Design review of the part built by this model. Coordinates are the model's own, in mm. A direction names the side the tool comes from. Coordinates: 2 decimals unless noted, no trailing zeros. Write each loop counter-clockwise with the first axis right and the second up, starting at its lowest first coordinate (ties: lowest second). Pieces come first, ordered by that corner, then holes. Notation, with made-up numbers: (69.5, 26) - (124.5, 26) arc R25 cw to (124.5, 51) - close; hole circle Ø1 at (-32, 84). An arc over 180 degrees is marked (long way). One line per item, written item: value.
from build123d import *

# Parameters (mm, degrees)
SKETCH_1_W          = 2
SKETCH_1_H          = 7
EXTRUDE_2_DEPTH     = 7
FILLET_1_R          = 3.5
SKETCH_2_R          = 1.55
CUT_EXTRUDE_1_DEPTH = 17.408839081
SKETCH_3_W          = 3.5
SKETCH_3_H          = 3
EXTRUDE_4_DEPTH     = 7
FILLET_2_R          = 3.5
SKETCH_4_R          = 1.5
CUT_EXTRUDE_2_DEPTH = 15.230249471
FILLET_3_R          = 3.5
FILLET_4_R          = 1.5
FILLET_5_R          = 0.8


# Some blends are built 0.0001 mm under size
with BuildPart() as part:
    # 草图1 → 凸台-拉伸2 (new body)
    with BuildSketch(Plane(origin=(0, 0, 0), x_dir=(1, 0, 0), z_dir=(0, 1, 0))):
        Polygon((-3.5, -3.5), (-3.5, 3.5), (-0.5, 3.5), (-0.5, 5.5), (-2.5, 5.5), (-5.5, 5.5), (-5.5, -5.5), (5.5, -5.5), (5.5, 5.5), (2.5, 5.5), (0.5, 5.5), (0.5, 3.5), (3.5, 3.5), (3.5, -3.5), align=None)
        with Locations((-1.5, 9)):
            Rectangle(SKETCH_1_W, SKETCH_1_H)
        with Locations((1.5, 9)):
            Rectangle(SKETCH_1_W, SKETCH_1_H)
    extrude(amount=EXTRUDE_2_DEPTH)

    # 圆角1
    fillet_1_edges = [part.edges().sort_by_distance(p)[0] for p in [
        (1.5, 7, -12.5),
        (1.5, 0, -12.5),
        (-1.5, 0, -12.5),
        (-1.5, 7, -12.5),
    ]]
    fillet(fillet_1_edges, radius=FILLET_1_R - 0.0001)  # a hair under: the kernel refuses the full size

    # 草图2 → 切除-拉伸1 (cut, through all)
    with BuildSketch(Plane(origin=(2.5, 0, 0), x_dir=(0, 0, -1), z_dir=(1, 0, 0))):
        with Locations((9, 3.5)):
            Circle(SKETCH_2_R)
    extrude(amount=-CUT_EXTRUDE_1_DEPTH, mode=Mode.SUBTRACT)

    # 草图3 → 凸台-拉伸4 (add)
    with BuildSketch(Plane.XY.offset(5.5)):
        with Locations((-1.75, 1.5)):
            Rectangle(SKETCH_3_W, SKETCH_3_H)
        with Locations((1.75, 1.5)):
            Rectangle(SKETCH_3_W, SKETCH_3_H)
    extrude(amount=EXTRUDE_4_DEPTH)

    # 圆角2
    fillet_2_edges = [part.edges().sort_by_distance(p)[0] for p in [
        (3.5, 1.5, 12.5),
        (-3.5, 1.5, 12.5),
    ]]
    fillet(fillet_2_edges, radius=FILLET_2_R - 0.0001)  # a hair under: the kernel refuses the full size

    # 草图4 → 切除-拉伸2 (cut, through all)
    with BuildSketch(Plane(origin=(0, 3, 0), x_dir=(1, 0, 0), z_dir=(0, 1, 0))):
        with Locations(Location((0, -9, 0), (0, 0, 180))):
            Circle(SKETCH_4_R)
    extrude(amount=-CUT_EXTRUDE_2_DEPTH, mode=Mode.SUBTRACT)

    # 圆角3
    # the kernel refuses this fillet: 3.5 mm, written as the material it adds along each edge
    with BuildSketch(Plane(origin=(3.5, 0, 5.5), x_dir=(1, 0, 0), z_dir=(0, 1, 0))) as fillet_3_piece_1:
        with BuildLine():
            CenterArc((3.5, -3.16227766), FILLET_3_R, 115.376933525, 64.623066475)
            Line((0, -3.16227766), (-0.07, -3.16227766))
            Line((-0.07, -3.16227766), (-0.07, 0))
            Line((-0.07, 0), (0, 0.07))
            ThreePointArc((0, 0.07), (1, 0.07), (1.97, 0.063245553))
            Line((1.97, 0.063245553), (2, 0))
        make_face()
    extrude(amount=3)
    with BuildSketch(Plane(origin=(-3.5, 3, 5.5), x_dir=(0, 0, 1), z_dir=(0, -1, 0))) as fillet_3_piece_2:
        with BuildLine():
            CenterArc((3.16227766, 3.5), FILLET_3_R, 205.376933525, 64.623066475)
            Line((0, 2), (-0.063245553, 1.97))
            ThreePointArc((-0.063245553, 1.97), (-0.07, 1), (-0.07, 0))
            Line((-0.07, 0), (0, -0.07))
            Line((0, -0.07), (3.16227766, -0.07))
            Line((3.16227766, -0.07), (3.16227766, 0))
        make_face()
    extrude(amount=3)

    # 圆角4
    fillet_4_edges = [part.edges().sort_by_distance(p)[0] for p in [
        (-2.5, 3.5, -5.5),
        (2.5, 3.5, -5.5),
    ]]
    fillet(fillet_4_edges, radius=FILLET_4_R)

    # 圆角5
    fillet_5_edges = [part.edges().sort_by_distance(p)[0] for p in [
        (4.041960108, 0, 6.791448967),
        (-4.041960108, 0, 6.791448967),
        (4.75, 0, -5.5),
        (4.75, 7, -5.5),
        (-2.939339828, 0, -5.939339828),
        (-2.939339828, 7, -5.939339828),
        (2.939339828, 0, -5.939339828),
        (2.939339828, 7, -5.939339828),
        (5.5, 0, 0),
        (-5.5, 0, 0),
        (-4.75, 0, -5.5),
        (2.5, 0, -8.00005),
        (2.5, 7, -8.00005),
        (2.5, 1.025096977, -11.474903023),
        (2.5, 5.974903023, -11.474903023),
        (-2.5, 7, -8.00005),
        (-2.5, 0, -8.00005),
        (-4.75, 7, -5.5),
        (-2.5, 5.974903023, -11.474903023),
        (-2.5, 1.025096977, -11.474903023),
        (-5.5, 7, 0),
        (0, 7, 5.5),
        (5.5, 7, 0),
        (3.5, 0, 8.83118883),
        (-3.5, 0, 8.83118883),
        (-2.474903023, 0, 11.474903023),
        (2.474903023, 0, 11.474903023),
    ]]
    fillet(fillet_5_edges, radius=FILLET_5_R)


solid = part.part
1. Consider section B-B, the plane x = -0.75. Give the number of separate pieces and of enclosed holes in the cut face, then the cut area to 3 significant figures.
Answer block:
separate pieces: 3
enclosed holes: 1
area: 76.9 mm^2
2. Consider section A-A, the plane z = -3.75. Write out the cut boundary in (x, y).
Answer block:
outline: (-5.5, 0.8) arc R0.8 ccw to (-4.7, 0) - (-0.5, 0) - (-0.5, 7) - (-4.7, 7) arc R0.8 ccw to (-5.5, 6.2) - close; (0.5, 0) - (4.7, 0) arc R0.8 ccw to (5.5, 0.8) - (5.5, 6.2) arc R0.8 ccw to (4.7, 7) - (0.5, 7) - close
3. For faces 4 (the face through (0, 3, 3.5)), 5 (the face through (0, 3, 7)), 6 (the face through (2.5, 1.92, 11.45)), 7 (the face through (2.5, 5, -10)), 8 (the face through (0.5, 3, -7)), list the 3-axis set-ups (+Z, -Z, +X, -X, +Y, -Y) from which the entire face can be reached by the end or side of a thin tool; tool diameter is ignored.
Answer block:
face 4: +Y, -Y
face 5: +Z, +X, -X, +Y
face 6: +Z, +X, +Y, -Y
face 7: -Z, +X, +Y, -Y
face 8: -Z, +Y, -Y
4. Consider section C-C, the plane z = 0.25. Write out the cut boundary in (x, y), then the cut area to 3 significant figures.
Answer block:
outline: (-5.5, 0.8) arc R0.8 ccw to (-4.7, 0) - (-3.5, 0) - (-3.5, 7) - (-4.7, 7) arc R0.8 ccw to (-5.5, 6.2) - close; (3.5, 0) - (4.7, 0) arc R0.8 ccw to (5.5, 0.8) - (5.5, 6.2) arc R0.8 ccw to (4.7, 7) - (3.5, 7) - close
area: 27.5 mm^2
5. Wall thickness on line 1 along Y through (x, z) = (-1, -9); line 2 along X through (y, z) = (2.75, 3); line 3 along Z through (x, y) = (0, 1): over which ranges is each line inside the solid? List them lowest first.
Answer block:
line 1: y = 0 to 1.95, 5.05 to 7
line 2: x = -5.5 to -3.5, 3.5 to 5.5
line 3: z = 3.5 to 7.5, 10.5 to 12.5
6. Insertion check: pin 1 Ø5.5 at (x, z) = (2, 8.5) entering from +Y; pin 2 Ø4 at (y, z) = (2.5, -10) entering from -X; pin 3 Ø3.5 at (x, y) = (1.5, 5) entering from +Z; pin 4 Ø1.9 at (y, z) = (3.5, -9) entering from +X. Each pin has a flat end and moves straight along its axis. Give the tip position at first contact, or say it passes through.
Answer block:
pin 1: stops at y = 3
pin 2: stops at x = -2.5
pin 3: stops at z = 5.5
pin 4: passes through
7. Mouldability with a two-part tool opening along X and no side actions: class faces 1 (the face through (-1.486, 1.987, -8.664)), 2 (the face through (4.057, 1.885, 6.768)), 3 (the face through (-3.5, 3, 0)) as released by +X, released by -X, zero draft, split by the parting line, or undercut.
Answer block:
face 1: zero draft
face 2: released by +X
face 3: undercut
